Verification items for the finished model (mm, model axes). A direction names the side the tool comes from. Coordinates: 2 decimals unless noted, no trailing zeros. Order: outer loops, then holes, each group sorted by start corner. A loop starts at its lowest first (then second) coordinate and runs counter-clockwise, first axis right, second up. Notation, with made-up numbers: M 2,-7 L 39,-7 A16 ccw 39,-1 Z; hole C -35.75,35 d5. An arc over 180 degrees is marked long. Answer as a JSON object with one key per item and string values. Group by question number.
(1) Cross-section at C-C (y = 93.5). Enter the section's corners in (x, z), plus the area to 3 significant figures.
(2) Cross-section at B-B (y = 118). Enter the section's corners in (x, z).
(3) Cross-section at A-A (z = -3). Enter the section's corners in (x, y).
(4) Access from +Z, -Z, +X, -X, +Y, -Y to the whole of each face (thin tool, end or side, straight path). Record for faces 4 (the face through (70.5, 104, 3)), 5 (the face through (34, 115, 10.8)), 6 (the face through (68, 98, 10.6)).
(5) Mould release check, pull along X, two halves, no side actions. Record for faces 1 (the face through (33, 110, 17)), 2 (the face through (-0.815, 114.774, 19.443)), 3 (the face through (1.6, 103, -3)): released by +X, released by -X, zero draft, split by the parting line, or undercut.
(6) Gauge pin test, flat ends, axial feed: pin 1 Ø1.3 at (x, y) = (0, 107) entering from +Z; pin 2 Ø1.6 at (x, y) = (65.5, 98.5) entering from -Z; pin 3 Ø0.8 at (x, y) = (67.5, 98.5) entering from -Z. Record the tip position at first contact, or that the pin passes through.
(7) Material ranges on line 1 (X direction, y = 119, z = 1); line 2 (X direction, y = 117, z = 9); line 3 (Z direction, x = 51.5, y = 100.5), recorded low to high.
(8) Cross-section at D-D (x = 22). Enter the section's corners in (y, z).
from build123d import *

# Parameters (mm, degrees)
EXTRUDE036_DEPTH                     = 100
EXTRUDE035_DEPTH                     = 2
EXTRUDE035_ONTO_SKETCH048_ROLL_ANGLE = 90
BOX016_W                             = 80
BOX016_H                             = 28
BOX016_DEPTH                         = 30
EXTRUDE034_DEPTH                     = 35.5
EXTRUDE034_ONTO_SKETCH047_ROLL_ANGLE = 90


with BuildPart() as round_cut:
    # Sketch049 → Extrude036 (new body)
    with BuildSketch(Plane.YZ.offset(-14)):
        with BuildLine():
            Line((100, 23.2), (100, 26.2))
            Line((100, 26.2), (133, 26.2))
            Line((133, 26.2), (133, -6.8))
            Line((133, -6.8), (130, -6.8))
            Line((130, -6.8), (130, 3.2))
            ThreePointArc((130, 3.2), (124.142136, 17.342136), (110, 23.2))
            Line((100, 23.2), (110, 23.2))
        make_face()
    extrude(amount=EXTRUDE036_DEPTH)


with BuildPart() as extrude035:
    # Sketch048 as drawn → Extrude035 (new)
    with BuildSketch(Plane.XY):
        with BuildLine():
            Line((-2.5, 14.2), (-2.5, -4.1))
            ThreePointArc((-2.5, -4.1), (0.136039, -10.463961), (6.5, -13.1))
            Line((6.5, -13.1), (61.5, -13.1))
            ThreePointArc((61.5, -13.1), (67.863961, -10.463961), (70.5, -4.1))
            Line((70.5, -4.1), (70.5, 14.2))
            ThreePointArc((70.5, 14.2), (67.863961, 20.563961), (61.5, 23.2))
            Line((6.5, 23.2), (61.5, 23.2))
            ThreePointArc((6.5, 23.2), (0.136039, 20.563961), (-2.5, 14.2))
        make_face()
    extrude(amount=-EXTRUDE035_DEPTH)


with BuildPart() as extrude035_1:
    # Extrude035 onto Sketch048 roll: moved
    add(extrude035.part.rotate(Axis((0, 0, 0), (1, 0, 0)), EXTRUDE035_ONTO_SKETCH048_ROLL_ANGLE))


with BuildPart() as extrude035_2:
    # Extrude035 onto Sketch048 placement: moved
    add(extrude035_1.part.moved(Location((0, 120, 0))))


with BuildPart() as extrude035_3:
    # Extrude035 placement: moved
    add(extrude035_2.part.moved(Location((0, 0.5, 0))))


with BuildPart() as cube004:
    # Box016 → Box016 (new body)
    with BuildSketch(Plane(origin=(-5, 82, 10.6), x_dir=(1, 0, 0), z_dir=(0, 0, 1))):
        with Locations((40, 14)):
            Rectangle(BOX016_W, BOX016_H)
    extrude(amount=BOX016_DEPTH)


with BuildPart() as cut012:
    # Sketch047 as drawn → Extrude034 (new)
    with BuildSketch(Plane.XY):
        with BuildLine():
            Line((-2.5, 14.2), (-2.5, -4.1))
            ThreePointArc((-2.5, -4.1), (0.136039, -10.463961), (6.5, -13.1))
            Line((6.5, -13.1), (61.5, -13.1))
            ThreePointArc((61.5, -13.1), (67.863961, -10.463961), (70.5, -4.1))
            Line((70.5, -4.1), (70.5, 14.2))
            ThreePointArc((70.5, 14.2), (67.863961, 20.563961), (61.5, 23.2))
            Line((6.5, 23.2), (61.5, 23.2))
            ThreePointArc((6.5, 23.2), (0.136039, 20.563961), (-2.5, 14.2))
        make_face()
        with BuildLine():
            Line((1.6, 1.2), (-1, 1.2))
            Line((-1, 1.2), (-1, -0.1))
            Line((-1, -0.1), (1.6, -0.1))
            Line((1.6, -0.1), (1.6, -6.1))
            ThreePointArc((1.6, -6.1), (3.064466, -9.635534), (6.6, -11.1))
            Line((6.6, -11.1), (61.4, -11.1))
            ThreePointArc((61.4, -11.1), (64.935534, -9.635534), (66.4, -6.1))
            Line((66.4, -0.1), (66.4, -6.1))
            Line((69, -0.1), (66.4, -0.1))
            Line((69, 1.2), (69, -0.1))
            Line((66.4, 1.2), (69, 1.2))
            Line((66.4, 5.4), (66.4, 1.2))
            Line((64.4, 5.4), (66.4, 5.4))
            Line((64.4, 7.4), (64.4, 5.4))
            Line((66.4, 7.4), (64.4, 7.4))
            Line((66.4, 10.6), (66.4, 7.4))
            Line((66.4, 10.6), (66.4, 10.8))
            Line((66.4, 10.8), (64.5, 10.8))
            Line((64.5, 10.8), (3.5, 10.8))
            Line((1.6, 10.8), (3.5, 10.8))
            Line((1.6, 10.6), (1.6, 10.8))
            Line((1.6, 10.6), (1.6, 7.4))
            Line((1.6, 7.4), (3.5, 7.4))
            Line((3.5, 7.4), (1.6, 1.2))
        make_face(mode=Mode.SUBTRACT)
    extrude(amount=EXTRUDE034_DEPTH)


with BuildPart() as cut012_1:
    # Extrude034 onto Sketch047 roll: moved
    add(cut012.part.rotate(Axis((0, 0, 0), (1, 0, 0)), EXTRUDE034_ONTO_SKETCH047_ROLL_ANGLE))


with BuildPart() as cut012_2:
    # Extrude034 onto Sketch047 placement: moved
    add(cut012_1.part.moved(Location((0, 120, 0))))


with BuildPart() as cut012_3:
    # Extrude034 placement: moved
    add(cut012_2.part.moved(Location((0, 1.5, 0))))

    # Cut011: cut Cube004
    add(cube004.part, mode=Mode.SUBTRACT)

    # Fusion020: union Extrude035
    add(extrude035_3.part)

    # Cut012: cut round_cut
    add(round_cut.part, mode=Mode.SUBTRACT)


solid = cut012_3.part
Taken from the geometry:
{
 "1": {"outline": "M -2.5,-4.1 A9 ccw 6.5,-13.1 L 61.5,-13.1 A9 ccw 70.5,-4.1 L 70.5,10.6 L 66.4,10.6 L 66.4,7.4 L 64.4,7.4 L 64.4,5.4 L 66.4,5.4 L 66.4,1.2 L 69,1.2 L 69,-0.1 L 66.4,-0.1 L 66.4,-6.1 A5 cw 61.4,-11.1 L 6.6,-11.1 A5 cw 1.6,-6.1 L 1.6,-0.1 L -1,-0.1 L -1,1.2 L 1.6,1.2 L 3.5,7.4 L 1.6,7.4 L 1.6,10.6 L -2.5,10.6 Z", "area": "303 mm²"},
 "2": {"outline": "M -2.5,-4.1 A9 ccw 6.5,-13.1 L 61.5,-13.1 A9 ccw 70.5,-4.1 L 70.5,14.2 A9 ccw 66.72,21.53 L 1.28,21.53 A9 ccw -2.5,14.2 Z; hole M -1,-0.1 L 1.6,-0.1 L 1.6,-6.1 A5 ccw 6.6,-11.1 L 61.4,-11.1 A5 ccw 66.4,-6.1 L 66.4,-0.1 L 69,-0.1 L 69,1.2 L 66.4,1.2 L 66.4,5.4 L 64.4,5.4 L 64.4,7.4 L 66.4,7.4 L 66.4,10.8 L 1.6,10.8 L 1.6,7.4 L 3.5,7.4 L 1.6,1.2 L -1,1.2 Z"},
 "3": {"outline": "M -2.5,86 L 1.6,86 L 1.6,120.5 L 66.4,120.5 L 66.4,86 L 70.5,86 L 70.5,122.5 L -2.5,122.5 Z"},
 "4": {"face 4": "+Z, -Z, +X, +Y, -Y", "face 5": "-Y", "face 6": "+Z, +X, -X, -Y"},
 "5": {"face 1": "zero draft", "face 2": "released by -X", "face 3": "undercut"},
 "6": {"pin 1": "stops at z = 10.6", "pin 2": "stops at z = -12.51", "pin 3": "stops at z = -11.15"},
 "7": {"line 1": "x = -2.5 to -1, 69 to 70.5", "line 2": "x = -2.5 to 1.6, 66.4 to 70.5", "line 3": "z = -13.1 to -11.1"},
 "8": {"outline": "M 86,-13.1 L 122.5,-13.1 L 122.5,18.81 A20 ccw 110,23.2 L 110,10.8 L 120.5,10.8 L 120.5,-11.1 L 86,-11.1 Z"}
}
